Check sheet for the modelled part. Datum: model origin and axes. Units: mm. A direction names the side the tool comes from. Coordinates: 2 decimals unless noted, no trailing zeros. Loops run counter-clockwise (first coordinate to the right, second up) from the corner with the lowest first, then second, coordinate; pieces in that order, holes last. Notation, with made-up numbers: M 44,45.25 L 95,45.25 A29 ccw 95,72.25 Z; hole C 66.25,5 d8. An arc over 180 degrees is marked long. Use CSV: the item, a comma, the result in double quotes. Start each with the question number.
(1) Scan lines: line 1 (Z direction, x = -35, y = -63); line 2 (X direction, y = -580, z = 36.5). Record each from-to range of solid material in increasing order.
(2) Section check A-A on z = -26.5. Record the cut outline in (x, y).
(3) Set-up check for faces 1 (the flat face through (0, -394, 40)), 2 (the flat face through (-37, -394, -1)): record each of +Z, -Z, +X, -X, +Y, -Y from which the full face is reachable in a straight line by a thin tool's end or side.
(4) Section check C-C on x = -16. Record the cut outline in (y, z).
(5) Section check B-B on y = -724.5. Record the cut outline in (x, z).
(6) Draft check along X on faces 3 (the flat face through (0, -394, -40)), 4 (the flat face through (40, -394, 0)), 5 (the flat face through (-1, -394, -37)), 6 (the flat face through (-40, -394, 0)). Enter one of: pulls with the +X half, pulls with the -X half, needs draft (parallel to the pull), parting line crosses it, or undercut.
from build123d import *

# Parameters (mm, degrees)
F0_W     = 80
F0_H     = 80
F0_W_2   = 74
F0_H_2   = 74
F1_DEPTH = 800
F2_R     = 5


with BuildPart() as f1:
    # F0 (on Front) → F1 (new body)
    with BuildSketch(Plane.XZ):
        Rectangle(F0_W, F0_H)
        Rectangle(F0_W_2, F0_H_2, mode=Mode.SUBTRACT)
    extrude(amount=F1_DEPTH)

    # F2
    f2_edges = [f1.edges().sort_by_distance(p)[0] for p in [
        (40, -400, 40),
        (-40, -400, 40),
        (40, -400, -40),
        (-40, -400, -40),
    ]]
    fillet(f2_edges, radius=F2_R)


solid = f1.part
Outcome:
1,line 1,"z = -40 to -37, 37 to 40"
1,line 2,"x = -39.77 to -37, 37 to 39.77"
2,outline,"M -40,-800 L -37,-800 L -37,0 L -40,0 Z; M 37,-800 L 40,-800 L 40,0 L 37,0 Z"
3,face 1,"+Z, +X, -X, +Y, -Y"
3,face 2,"+Y, -Y"
4,outline,"M -800,-40 L 0,-40 L 0,-37 L -800,-37 Z; M -800,37 L 0,37 L 0,40 L -800,40 Z"
5,outline,"M -40,-35 A5 ccw -35,-40 L 35,-40 A5 ccw 40,-35 L 40,35 A5 ccw 35,40 L -35,40 A5 ccw -40,35 Z; hole M -37,-37 L 37,-37 L 37,37 L -37,37 Z"
6,face 3,"needs draft"
6,face 4,"pulls with the +X half"
6,face 5,"undercut"
6,face 6,"pulls with the -X half"
